CAD build for the part. Positions are in the model's coordinates, mm. A direction names the side the tool comes from. Give positions to 0.01 mm unless a question says otherwise; leave off trailing zeros. Loops run counter-clockwise (first coordinate to the right, second up) from the corner with the lowest first, then second, coordinate; pieces in that order, holes last.
Item 1: Saw through at C-C on x = 0. Give the cut face in (y, z), plus the area to 3 significant figures.
Item 2: Drop flat-ended pins along their axis: P1, Ø6, axis at x = 25, z = -12.5, coming from the +Y side; P2, Ø3, axis at y = -1, z = -35, coming from the -X side; P3, Ø3, axis at x = -25, y = 0, coming from the +Z side. Give the stop position or say it passes through.
Item 3: Probe probe 1 along X at (y, z) = (-0.95, 0); probe 2 along X at (y, z) = (-0.5, 11); probe 3 along Z at (x, y) = (-21, -1.55). List the from-to ranges inside material, lowest first.
Item 4: Saw through at A-A on z = 28. Give the cut face in (x, y).
Item 5: Saw through at B-B on z = 0. Give the cut face in (x, y).
Item 6: Saw through at D-D on x = -19. Give the cut face in (y, z).
Item 7: Which spindle directions (+Z, -Z, +X, -X, +Y, -Y) get a long thin tool onto all of the face, cutting with end or side? Do faces 1 (the flat face through (0, 2.5, 3)), 2 (the cylindrical face through (-4.868, 0.035, -6.349)), 3 (the flat face through (-27.12, -0.98, -15.42)), 4 (the flat face through (25.76, 0.45, -17.71)). Say none if no direction does.
Item 8: Mould opens along Z. For faces 5 (the cylindrical face through (-22.21, 0.04, 53.58)), 6 (the flat face through (-28.222, 0.448, -13.454)), 7 (the flat face through (-0.21, 0.98, 31.19)), 8 (the flat face through (-30, 2.5, 47)) say: released by +Z, released by -Z, zero draft, split by the parting line, or undercut.
from build123d import *

# Parameters (mm, degrees)
SKETCH7_R                = 58
SKETCH7_R_2              = 55.5
BOSS_EXTRUDE4_DEPTH      = 2.5
BOSS_EXTRUDE5_REACH      = 84.062
BOSS_EXTRUDE5_END_RADIUS = 55.5
SKETCH2_R                = 8
BOSS_EXTRUDE6_DEPTH      = 2.5
CIRPATTERN5_COUNT        = 3
CUT_EXTRUDE2_DEPTH       = 10


with BuildPart() as part:
    # Sketch7 → Boss-Extrude4 (new, symmetric)
    with BuildSketch(Plane(origin=(0, 0, 0), x_dir=(1, 0, 0), z_dir=(0, 1, 0))):
        with Locations(Location((0, 0, 0), (0, 0, 270))):
            Circle(SKETCH7_R)
        with Locations(Location((0, 0, 0), (0, 0, 270))):
            Circle(SKETCH7_R_2, mode=Mode.SUBTRACT)
    extrude(amount=BOSS_EXTRUDE4_DEPTH, both=True)

    # Boss-Extrude5: up to this cylinder (the profile starts inside it)
    boss_extrude5_end = Plane(origin=(0, 0, 0), z_dir=(0, -1, 0)) * Cylinder(BOSS_EXTRUDE5_END_RADIUS, 280.124, mode=Mode.PRIVATE)
    # Sketch1 → Boss-Extrude5 (add, up to the surface)
    with BuildSketch(Plane.XY, mode=Mode.PRIVATE) as boss_extrude5_sk1:
        Polygon((2.288371205, 1.418928197), (2.63566756, -0.550687309), (-2.288371205, -1.418928197), (-2.63566756, 0.550687309), align=None)
    boss_extrude5_tool1 = extrude(boss_extrude5_sk1.sketch, amount=BOSS_EXTRUDE5_REACH, mode=Mode.PRIVATE) & boss_extrude5_end
    boss_extrude5 = boss_extrude5_tool1.solids().sort_by_distance((0, 0, 0))[0]
    add(boss_extrude5)

    # Sketch2 → Boss-Extrude6 (add, symmetric)
    with BuildSketch(Plane(origin=(0, 0, 0), x_dir=(1, 0, 0), z_dir=(0, 1, 0))):
        with Locations(Location((0, 0, 0), (0, 0, 270))):
            Circle(SKETCH2_R)
    extrude(amount=BOSS_EXTRUDE6_DEPTH, both=True)

    # CirPattern5: Boss-Extrude5 ×3 about axis
    cirpattern5_axis = Axis((0, 0, 0), (0, 1, 0))
    for i in range(1, CIRPATTERN5_COUNT):
        add(boss_extrude5.rotate(cirpattern5_axis, i * 360 / CIRPATTERN5_COUNT))

    # Sketch9 → Cut-Extrude2 (cut)
    with BuildSketch(Plane(origin=(0, 2.5, 0), x_dir=(1, 0, 0), z_dir=(0, 1, 0))):
        with BuildLine():
            ThreePointArc((-4.399803026, -5.444422222), (-7, 0), (-4.399803026, 5.444422222))
            ThreePointArc((-4.399803026, 5.444422222), (0, 2.3333), (4.399803026, 5.444422222))
            ThreePointArc((4.399803026, 5.444422222), (7, 0), (4.399803026, -5.444422222))
            ThreePointArc((4.399803026, -5.444422222), (0, -2.3333), (-4.399803026, -5.444422222))
        make_face()
    extrude(amount=-CUT_EXTRUDE2_DEPTH, mode=Mode.SUBTRACT)


solid = part.part
Results below:
1. outline: (-2.5, -58) - (2.5, -58) - (2.5, -55.5) - (-2.5, -55.5) - close; (-2.5, -8) - (2.5, -8) - (2.5, -2.33) - (-2.5, -2.33) - close; (-2.5, 2.33) - (2.5, 2.33) - (2.5, 8) - (1.02, 8) - (1.02, 55.5) - (2.5, 55.5) - (2.5, 58) - (-2.5, 58) - (-2.5, 55.5) - (-1.02, 55.5) - (-1.02, 8) - (-2.5, 8) - close
1. area: 178 mm2
2. P1: stops at y = 1.25
2. P2: stops at x = -47.35
2. P3: stops at z = 53.03
3. probe 1: x = -58 to -55.5, -8 to -7, 7 to 8, 55.5 to 58
3. probe 2: x = -56.95 to -54.4, -2.45 to 2.63, 54.4 to 56.95
3. probe 3: z = -54.06 to -51.37, 51.37 to 54.06
4. outline: (-50.79, -2.5) - (-47.92, -2.5) - (-47.92, 2.5) - (-50.79, 2.5) - close; (-2.64, 0.55) - (-2.29, -1.42) - (2.64, -0.55) - (2.29, 1.42) - close; (47.92, -2.5) - (50.79, -2.5) - (50.79, 2.5) - (47.92, 2.5) - close
5. outline: (-58, -2.5) - (-55.5, -2.5) - (-55.5, 2.5) - (-58, 2.5) - close; (-8, -2.5) - (-7, -2.5) - (-7, 2.5) - (-8, 2.5) - close; (7, -2.5) - (8, -2.5) - (8, 2.5) - (7, 2.5) - close; (55.5, -2.5) - (58, -2.5) - (58, 2.5) - (55.5, 2.5) - close
6. outline: (-2.5, -54.8) - (2.5, -54.8) - (2.5, -52.15) - (-2.5, -52.15) - close; (-2.5, 52.15) - (2.5, 52.15) - (2.5, 54.8) - (-2.5, 54.8) - close; (-1.42, -13.61) - (0.55, -14.01) - (1.42, -8.33) - (-0.55, -7.93) - close
7. face 1: +Z, -Z, +X, -X, +Y
7. face 2: none
7. face 3: -Y
7. face 4: +Y
8. face 5: split by the parting line
8. face 6: undercut
8. face 7: undercut
8. face 8: zero draft
